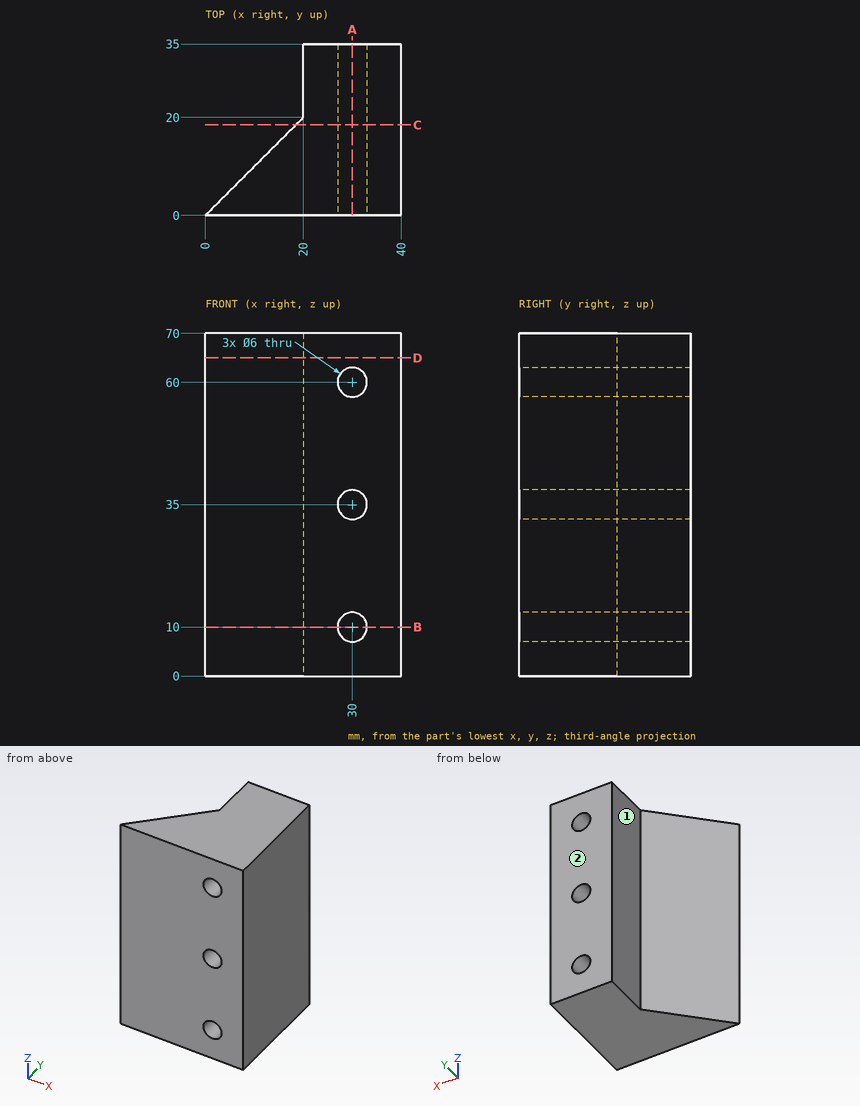
Answer from the drawing. Dimensions are ordinates in mm from the lowest x, y and z of the part. A direction names the side the tool comes from. Give positions to 0.01 mm unless a question says otherwise; leave off trailing zeros. Loops run counter-clockwise (first coordinate to the right, second up) from the corner with the lowest first, then second, coordinate; pieces in that order, holes last.
Item 1: For the marked faces 1 and 2, determine the directions among +Z, -Z, +X, -X, +Y, -Y from which every point of the face is accessible in a straight line to the end or side of a thin tool.
Item 2: Each of these flat-tipped pins is pushed along its axis until it touches: pin 1 Ø3.5 at (x, z) = (30, 35) entering from -Y; pin 2 Ø4 at (y, z) = (14.5, 38.5) entering from -X; pin 3 Ø6 at (x, z) = (8, 21) entering from +Y; pin 4 Ø16.5 at (y, z) = (26.5, 38) entering from -X. Where does it stop, or does it pass through?
Item 3: Find the intervals of material crossed by line 1 along Z through (x, y) = (30, 7); line 2 along Z through (x, y) = (29, 15); line 3 along X through (y, z) = (21.5, 35), in increasing order.
Item 4: The part is cut by section D-D (z = 65). Write down the section's boundary in (x, y), and give its area (3 significant figures).
Item 5: The part is cut by section A-A (x = 30). Write down the section's boundary in (y, z).
Item 6: The part is cut by section B-B (z = 10). Write down the section's boundary in (x, y).
Item 7: The part is cut by section C-C (y = 18.5). Write down the section's boundary in (x, z).
Taken from the geometry:
1. face 1: +Z, -Z, -X, +Y
1. face 2: +Z, -Z, +X, -X, +Y
2. pin 1: passes through
2. pin 2: stops at x = 12.5
2. pin 3: stops at y = 11
2. pin 4: stops at x = 18.25
3. line 1: z = 0 to 7, 13 to 32, 38 to 57, 63 to 70
3. line 2: z = 0 to 7.17, 12.83 to 32.17, 37.83 to 57.17, 62.83 to 70
3. line 3: x = 20 to 27, 33 to 40
4. outline: (0, 0) - (40, 0) - (40, 35) - (20, 35) - (20, 20) - close
4. area: 900 mm2
5. outline: (0, 0) - (35, 0) - (35, 7) - (0, 7) - close; (0, 13) - (35, 13) - (35, 32) - (0, 32) - close; (0, 38) - (35, 38) - (35, 57) - (0, 57) - close; (0, 63) - (35, 63) - (35, 70) - (0, 70) - close
6. outline: (0, 0) - (27, 0) - (27, 35) - (20, 35) - (20, 20) - close; (33, 0) - (40, 0) - (40, 35) - (33, 35) - close
7. outline: (18.5, 0) - (40, 0) - (40, 70) - (18.5, 70) - close; hole circle Ø6 at (30, 10); hole circle Ø6 at (30, 35); hole circle Ø6 at (30, 60)
